Answer from the drawing. Dimensions are ordinates in mm from the lowest x, y and z of the part. A direction names the side the tool comes from. Round coordinates to 2 decimals unless told otherwise and drop trailing zeros. Write each loop counter-clockwise with the first axis right and the second up, starting at its lowest first coordinate (ties: lowest second). Pieces come first, ordered by that corner, then holes.
1. A tool of negligible diameter and unlimited length cuts with its end or side. For the marked faces 1, 2 and 3, from which of +Z, -Z, +X, -X, +Y, -Y can it reach the whole face along a straight path? Write none if from no direction.
2. Flat-ended cylindrical pins translate along their axes: pin 1 Ø1.1 at (y, z) = (8, 1.5) entering from +X; pin 2 Ø1.5 at (y, z) = (8.5, 2) entering from -X; pin 3 Ø1.5 at (y, z) = (5, 2.5) entering from +X. Find the tip coordinate at first contact, or state that the pin passes through.
3. Find section A-A (z = 0.6). Write down the section's boundary in (x, y), and give its area (3 significant figures).
4. Find section B-B (y = 8.5). Write down the section's boundary in (x, z).
5. Straight lines are drawn through the part: probe 1 along X at (y, z) = (5.75, 1.85); probe 2 along Y at (x, z) = (3, 0.55); probe 3 along Y at (x, z) = (5.5, 2.8). For each, find the intervals that lie inside material, in ascending order.
6. Find section C-C (x = 18.5). Write down the section's boundary in (y, z), and give its area (3 significant figures).
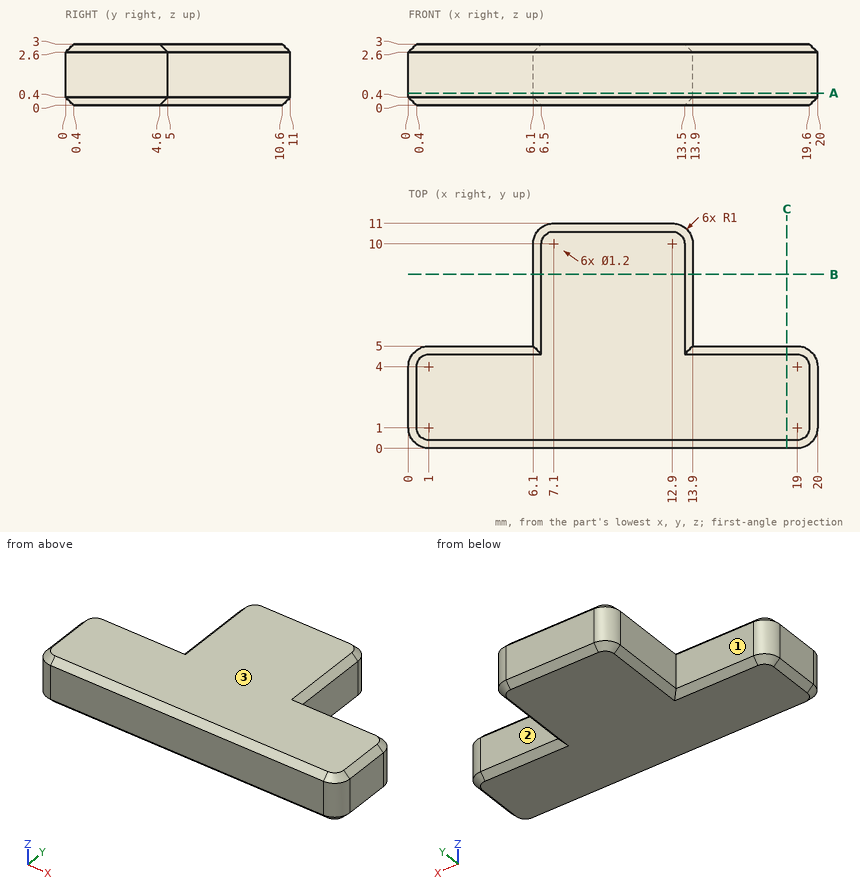
Worked answers:
1. face 1: +Z, -Z, -X, +Y
1. face 2: +Z, -Z, +X, +Y
1. face 3: +Z, +X, -X, +Y, -Y
2. pin 1: stops at x = 13.9
2. pin 2: stops at x = 6.1
2. pin 3: stops at x = 19.97
3. outline: (0, 1) arc R1 ccw to (1, 0) - (19, 0) arc R1 ccw to (20, 1) - (20, 4) arc R1 ccw to (19, 5) - (13.9, 5) - (13.9, 10) arc R1 ccw to (12.9, 11) - (7.1, 11) arc R1 ccw to (6.1, 10) - (6.1, 5) - (1, 5) arc R1 ccw to (0, 4) - close
3. area: 146 mm2
4. outline: (6.1, 0.4) - (6.5, 0) - (13.5, 0) - (13.9, 0.4) - (13.9, 2.6) - (13.5, 3) - (6.5, 3) - (6.1, 2.6) - close
5. probe 1: x = 6.1 to 13.9
5. probe 2: y = 0 to 5
5. probe 3: y = 0.2 to 4.8
6. outline: (0, 0.4) - (0.4, 0) - (4.6, 0) - (5, 0.4) - (5, 2.6) - (4.6, 3) - (0.4, 3) - (0, 2.6) - close
6. area: 14.7 mm2
